from build123d import *

# Parameters (mm, degrees)
SKETCH_1_R               = 60
SKETCH_1_R_2             = 10
EXTRUDE_1_DEPTH          = 60
CUT_EXTRUDE_1_DEPTH      = 60
PATTERN_CIRCULAR_1_COUNT = 6
FILLET_1_R               = 5


with BuildPart() as part:
    # Sketch 1 → Extrude 1 (new body)
    with BuildSketch(Plane.XY):
        Circle(SKETCH_1_R)
        Circle(SKETCH_1_R_2, mode=Mode.SUBTRACT)
    extrude(amount=-EXTRUDE_1_DEPTH)

    # Sketch 2 → Cut-Extrude 1 (cut)
    with BuildSketch(Plane.XY):
        with BuildLine():
            Line((-8.682408883, 49.240387651), (-3.472963553, 19.69615506))
            ThreePointArc((-3.472963553, 19.69615506), (0, 20), (3.472963553, 19.69615506))
            Line((3.472963553, 19.69615506), (8.682408883, 49.240387651))
            ThreePointArc((8.682408883, 49.240387651), (0, 50), (-8.682408883, 49.240387651))
        make_face()
    cut_extrude_1 = extrude(amount=-CUT_EXTRUDE_1_DEPTH, mode=Mode.SUBTRACT)

    # Pattern Circular 1: Cut-Extrude 1 ×6 about axis
    pattern_circular_1_axis = Axis((0, 0, 0), (0, 0, 1))
    for i in range(1, PATTERN_CIRCULAR_1_COUNT):
        add(cut_extrude_1.rotate(pattern_circular_1_axis, i * 360 / PATTERN_CIRCULAR_1_COUNT), mode=Mode.SUBTRACT)

    # Fillet 1
    fillet_1_edges = [part.edges().sort_by_distance(p)[0] for p in [
        (-60, 0, 0),
        (-60, 0, -60),
    ]]
    fillet(fillet_1_edges, radius=FILLET_1_R)


solid = part.part
Could you check a few things on this model? Use its own coordinates, in mm. Give positions to 0.01 mm unless a question says otherwise; leave off trailing zeros. Order: outer loops, then holes, each group sorted by start corner. A loop starts at its lowest first (then second) coordinate and runs counter-clockwise, first axis right, second up. Notation, with made-up numbers: (28.25, 31) - (40.25, 31) arc R16 ccw to (40.25, 37) - close; hole circle Ø4 at (5.5, 4). An arc over 180 degrees is marked (long way). One line per question, with ' | ' between items. Start each with the question number.
Item 1: I want a section at C-C on z = -14.5. Write out the boundary of the cut face in (x, y).
Item 2: I'm going to push flat-ended pins straight in: pin 1 Ø4 at (y, z) = (22, -16) entering from -X; pin 2 Ø1 at (x, z) = (11, -42.5) entering from +Y; pin 3 Ø8 at (y, z) = (-7.5, -47) entering from -X. Where does each tip first touch, or does it pass through?
Item 3: I want a section at B-B on y = 0. Write out the boundary of the cut face in (x, z), then the cut area to 3 significant figures.
Item 4: I want a section at D-D on x = -30. Give the number of separate pieces and of enclosed holes in the cut face, then the cut area to 3 significant figures.
Item 5: I want a section at A-A on x = 0. Write out the boundary of the cut face in (y, z), then the cut area to 3 significant figures.
Item 6: I need wall thicknesses on probe 1 along Y at (x, z) = (-37, -8); probe 2 along Y at (x, z) = (43, -7.5); probe 3 along X at (y, z) = (29.5, -25.5). Which ranges of each line are inside material? Lowest first, please. Write a range as [from, to].
Verdict:
1) outline: circle Ø120 at (0, 0); hole (-46.98, -17.1) arc R50 ccw to (-38.3, -32.14) - (-15.32, -12.86) arc R20 cw to (-18.79, -6.84) - close; hole (-46.98, 17.1) - (-18.79, 6.84) arc R20 cw to (-15.32, 12.86) - (-38.3, 32.14) arc R50 ccw to start; hole circle Ø20 at (0, 0); hole (-8.68, -49.24) arc R50 ccw to (8.68, -49.24) - (3.47, -19.7) arc R20 cw to (-3.47, -19.7) - close; hole (-8.68, 49.24) - (-3.47, 19.7) arc R20 cw to (3.47, 19.7) - (8.68, 49.24) arc R50 ccw to start; hole (15.32, -12.86) - (38.3, -32.14) arc R50 ccw to (46.98, -17.1) - (18.79, -6.84) arc R20 cw to start; hole (15.32, 12.86) arc R20 cw to (18.79, 6.84) - (46.98, 17.1) arc R50 ccw to (38.3, 32.14) - close
2) pin 1: x = -56.57 | pin 2: y = 59.07 | pin 3: x = -59.9
3) outline: (-60, -55) arc R5 ccw to (-55, -60) - (-10, -60) - (-10, 0) - (-55, 0) arc R5 ccw to (-60, -5) - close; (10, -60) - (55, -60) arc R5 ccw to (60, -55) - (60, -5) arc R5 ccw to (55, 0) - (10, 0) - close | area: 5,980 mm^2
4) separate pieces: 3 | enclosed holes: 0 | area: 4,500 mm^2
5) outline: (-60, -55) arc R5 ccw to (-55, -60) - (-50, -60) - (-50, 0) - (-55, 0) arc R5 ccw to (-60, -5) - close; (-20, -60) - (-10, -60) - (-10, 0) - (-20, 0) - close; (10, -60) - (20, -60) - (20, 0) - (10, 0) - close; (50, -60) - (55, -60) arc R5 ccw to (60, -55) - (60, -5) arc R5 ccw to (55, 0) - (50, 0) - close | area: 2,380 mm^2
6) probe 1: [-47.23, -31.05], [-13.47, 13.47], [31.05, 47.23] | probe 2: [-41.84, -25.51], [-15.65, 15.65], [25.51, 41.84] | probe 3: [-52.25, -40.37], [-35.16, -5.2], [5.2, 35.16], [40.37, 52.25]
